```python
from build123d import *

# Parameters (mm, degrees)
ESQUISSE3_W             = 100
ESQUISSE3_H             = 100
BOSS_EXTRU_1_DEPTH      = 7.5
ESQUISSE4_W             = 5
ESQUISSE4_H             = 5
BOSS_EXTRU_2_DEPTH      = 5
ESQUISSE5_R             = 3.175
ESQUISSE5_R_2           = 1.42
ENL_V_MAT_EXTRU_1_DEPTH = 10
BOSS_EXTRU_3_DEPTH      = 82.5
ENL_V_MAT_EXTRU_2_DEPTH = 2
ESQUISSE8_W             = 17.977516738
ESQUISSE8_H             = 17.952716394
ESQUISSE8_H_2           = 18.02477834
ENL_V_MAT_EXTRU_3_DEPTH = 2
ESQUISSE10_W            = 2.045095135
ESQUISSE10_H            = 18.02477834
ESQUISSE10_H_2          = 17.952716394
ENL_V_MAT_EXTRU_4_DEPTH = 10


with BuildPart() as part:
    # Esquisse3 → Boss.-Extru.1 (new body)
    with BuildSketch(Plane.XY):
        Rectangle(ESQUISSE3_W, ESQUISSE3_H)
    extrude(amount=-BOSS_EXTRU_1_DEPTH)

    # Esquisse4 → Boss.-Extru.2 (add)
    with BuildSketch(Plane(origin=(0, 0, -7.5), x_dir=(-1, 0, 0), z_dir=(0, 0, -1))):
        with Locations((-37.534911535, 47.5)):
            Rectangle(ESQUISSE4_W, ESQUISSE4_H)
        with Locations((37.5, 47.5)):
            Rectangle(ESQUISSE4_W, ESQUISSE4_H)
        with Locations((47.5, 37.5)):
            Rectangle(ESQUISSE4_W, ESQUISSE4_H)
        with Locations((47.5, -37.5)):
            Rectangle(ESQUISSE4_W, ESQUISSE4_H)
        with Locations((37.5, -47.5)):
            Rectangle(ESQUISSE4_W, ESQUISSE4_H)
        with Locations((-37.534911535, -47.5)):
            Rectangle(ESQUISSE4_W, ESQUISSE4_H)
        with Locations((-47.5, -33.92882297)):
            Rectangle(ESQUISSE4_W, ESQUISSE4_H)
        with Locations((-47.5, 37.5)):
            Rectangle(ESQUISSE4_W, ESQUISSE4_H)
    extrude(amount=BOSS_EXTRU_2_DEPTH)

    # Esquisse5 → Enlèv. mat.-Extru.1 (cut)
    with BuildSketch(Plane.XY):
        with Locations((-35, 19)):
            Circle(ESQUISSE5_R)
        with Locations((-39, -23.5)):
            Circle(ESQUISSE5_R)
        with Locations((-45.8, 45.8)):
            Circle(ESQUISSE5_R_2)
        with Locations((-45.8, -45.8)):
            Circle(ESQUISSE5_R_2)
        with Locations((45.8, -45.8)):
            Circle(ESQUISSE5_R_2)
        with Locations((45.8, 45.8)):
            Circle(ESQUISSE5_R_2)
        with Locations((-22, 20.1)):
            Circle(ESQUISSE5_R)
        with Locations((-22, -20.1)):
            Circle(ESQUISSE5_R)
    extrude(amount=-ENL_V_MAT_EXTRU_1_DEPTH, mode=Mode.SUBTRACT)

    # Esquisse6 → Boss.-Extru.3 (add)
    with BuildSketch(Plane.XY):
        Polygon((50, 0), (50, 39.1), (45, 39.1), (45, -39.1), (50, -39.1), align=None)
    extrude(amount=BOSS_EXTRU_3_DEPTH)

    # Esquisse7 → Enlèv. mat.-Extru.2 (cut)
    with BuildSketch(Plane.ZY.offset(-45)):
        Polygon((52.376358197, 39.1), (30.359102655, 39.1), (30.359102655, 31.140897345), (22.4, 31.09702268), (22.4, 9.07224434), (30.37224434, 9.07224434), (30.37224434, 1.1), (52.376358197, 1.1), (52.376358197, 9.123641803), (60.4, 9.07224434), (60.4, 31.09702268), (52.376358197, 31.076358197), align=None)
        Polygon((52.376358197, -1.1), (30.37224434, -1.1), (30.37224434, -9.07224434), (22.4, -9.07224434), (22.4, -31.079901273), (30.420098727, -31.079901273), (30.420098727, -39.1), (52.376358197, -39.1), (52.376358197, -31.076358197), (60.4, -31.076358197), (60.4, -9.123641803), (52.376358197, -9.123641803), align=None)
    extrude(amount=-ENL_V_MAT_EXTRU_2_DEPTH, mode=Mode.SUBTRACT)

    # Esquisse8 → Enlèv. mat.-Extru.3 (cut)
    with BuildSketch(Plane.ZY.offset(-45)):
        with Locations((69.388758369, -20.1)):
            Rectangle(ESQUISSE8_W, ESQUISSE8_H)
        with Locations((69.388758369, 20.08463351)):
            Rectangle(ESQUISSE8_W, ESQUISSE8_H_2)
    extrude(amount=-ENL_V_MAT_EXTRU_3_DEPTH, mode=Mode.SUBTRACT)

    # Esquisse10 → Enlèv. mat.-Extru.4 (cut)
    with BuildSketch(Plane.ZY.offset(-47)):
        with Locations((77.35496917, 20.08463351)):
            Rectangle(ESQUISSE10_W, ESQUISSE10_H)
        with Locations((77.35496917, -20.1)):
            Rectangle(ESQUISSE10_W, ESQUISSE10_H_2)
    extrude(amount=-ENL_V_MAT_EXTRU_4_DEPTH, mode=Mode.SUBTRACT)


solid = part.part
```
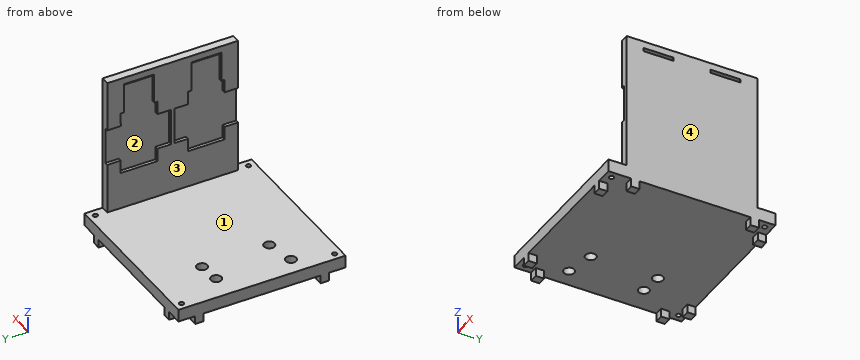
Verification items for the finished model (mm, model axes). Face numbers are marked on the shaded views. A direction names the side the tool comes from. Round coordinates to 2 decimals unless told otherwise and drop trailing zeros. Write each loop counter-clockwise with the first axis right and the second up, starting at its lowest first coordinate (ties: lowest second). Pieces come first, ordered by that corner, then holes. Notation, with made-up numbers: (71, -13) - (129, -13) arc R14 cw to (129, 13) - close; hole circle Ø6 at (8.5, 59.25). An arc over 180 degrees is marked (long way). Answer as a JSON object with one key per item and string values. Group by question number.
Q1. Go/stop test with flat-tipped pins: pin 1 Ø2.5 at (x, y) = (-45.8, -45.8) entering from +Z; pin 2 Ø1.5 at (x, z) = (-46.5, -9) entering from +Y; pin 3 Ø0.6 at (x, z) = (45.5, 25) entering from +Y; pin 4 Ø2.5 at (x, y) = (48.5, -19) entering from -Z. Record where each tip stops, or that it passes through.
Q2. Tool access check on the marked faces 3 and 4. Record the directions out of +Z, -Z, +X, -X, +Y, -Y that give a thin tool (end or side, any length) a straight path to the whole face; none if there is none.
Q3. Section check C-C, the plane z = 33.5. Enter the section's corners in (x, y).
Q4. Mould release check, pull along Y, two halves, no side actions. Record for the marked faces 1 and 2: released by +Y, released by -Y, zero draft, split by the parting line, or undercut.
Q5. Thickness scan on line 1 (Y direction, x = 45.8, z = -1.5); line 2 (X direction, y = -20, z = -2); line 3 (Y direction, x = 45, z = -5). Record the ranges inside material, lowest first.
Q6. Section check B-B, the plane y = -13. Enter the section's corners in (x, z).
Q7. Section check D-D, the plane y = 37. Enter the section's corners in (x, z), plus the area to 3 significant figures.
Q8. Section check A-A, the plane x = -22. Enter the section's corners in (y, z) (3 decimals).
Found:
{
 "1": {"pin 1": "passes through", "pin 2": "stops at y = 40", "pin 3": "stops at y = 39.1", "pin 4": "stops at z = -7.5"},
 "2": {"face 3": "+Z, -X, +Y, -Y", "face 4": "+Z, -Z, +X, +Y, -Y"},
 "3": {"outline": "(45, -1.1) - (47, -1.1) - (47, -39.1) - (50, -39.1) - (50, 39.1) - (47, 39.1) - (47, 1.1) - (45, 1.1) - close"},
 "4": {"face 1": "zero draft", "face 2": "undercut"},
 "5": {"line 1": "y = -50 to -47.22, -44.38 to 44.38, 47.22 to 50", "line 2": "x = -50 to -25.17, -18.83 to 50", "line 3": "y = -50 to -46.97, -44.63 to 44.63, 46.97 to 50"},
 "6": {"outline": "(-50, -7.5) - (50, -7.5) - (50, 76.33) - (47, 76.33) - (47, 22.4) - (45, 22.4) - (45, 0) - (-50, 0) - close; (45, 78.38) - (50, 78.38) - (50, 82.5) - (45, 82.5) - close"},
 "7": {"outline": "(-50, -12.5) - (-45, -12.5) - (-45, -7.5) - (45, -7.5) - (45, -12.5) - (50, -12.5) - (50, 82.5) - (45, 82.5) - (45, 52.38) - (47, 52.38) - (47, 30.36) - (45, 30.36) - (45, 0) - (-50, 0) - close", "area": "1,170 mm^2"},
 "8": {"outline": "(-50, -7.5) - (-23.275, -7.5) - (-23.275, 0) - (-50, 0) - close; (-16.925, -7.5) - (16.925, -7.5) - (16.925, 0) - (-16.925, 0) - close; (23.275, -7.5) - (50, -7.5) - (50, 0) - (23.275, 0) - close"}
}
